from build123d import *

# Parameters (mm, degrees)
CROQUIS1_W              = 100
CROQUIS1_H              = 100
SALIENTE_EXTRUIR1_DEPTH = 12.5
CROQUIS3_R              = 35.2
CORTAR_EXTRUIR1_DEPTH   = 9.2
CROQUIS4_R              = 25.5
CORTAR_EXTRUIR2_DEPTH   = 72.30666168
CROQUIS5_R              = 3.25
CORTAR_EXTRUIR3_DEPTH   = 72.807033082
MATRIZC1_COUNT          = 4
CROQUIS6_R              = 5.5
CORTAR_EXTRUIR4_DEPTH   = 6
MATRIZC2_COUNT          = 4


with BuildPart() as part:
    # Croquis1 → Saliente-Extruir1 (new body)
    with BuildSketch(Plane(origin=(0, 0, 0), x_dir=(1, 0, 0), z_dir=(0, 1, 0))):
        Rectangle(CROQUIS1_W, CROQUIS1_H)
    extrude(amount=SALIENTE_EXTRUIR1_DEPTH)

    # Croquis3 → Cortar-Extruir1 (cut)
    with BuildSketch(Plane.XZ):
        with Locations(Location((0, 0, 0), (0, 0, 270))):
            Circle(CROQUIS3_R)
    extrude(amount=-CORTAR_EXTRUIR1_DEPTH, mode=Mode.SUBTRACT)

    # Croquis4 → Cortar-Extruir2 (cut, through all)
    with BuildSketch(Plane.XZ.offset(-9.2)):
        with Locations(Location((0, 0, 0), (0, 0, 270))):
            Circle(CROQUIS4_R)
    extrude(amount=-CORTAR_EXTRUIR2_DEPTH, mode=Mode.SUBTRACT)

    # Croquis5 → Cortar-Extruir3 (cut, through all)
    with BuildSketch(Plane.XZ):
        with Locations(Location((-40, 40, 0), (0, 0, 270))):
            Circle(CROQUIS5_R)
    cortar_extruir3 = extrude(amount=-CORTAR_EXTRUIR3_DEPTH, mode=Mode.SUBTRACT)

    # MatrizC1: Cortar-Extruir3 ×4 about axis
    matrizc1_axis = Axis((0, 0, 0), (0, 1, 0))
    for i in range(1, MATRIZC1_COUNT):
        add(cortar_extruir3.rotate(matrizc1_axis, i * 360 / MATRIZC1_COUNT), mode=Mode.SUBTRACT)

    # Croquis6 → Cortar-Extruir4 (cut)
    with BuildSketch(Plane(origin=(0, 12.5, 0), x_dir=(1, 0, 0), z_dir=(0, 1, 0))):
        with Locations(Location((-40, 40, 0), (0, 0, 270))):
            Circle(CROQUIS6_R)
    cortar_extruir4 = extrude(amount=-CORTAR_EXTRUIR4_DEPTH, mode=Mode.SUBTRACT)

    # MatrizC2: Cortar-Extruir4 ×4 about axis
    matrizc2_axis = Axis((0, 0, 0), (0, 1, 0))
    for i in range(1, MATRIZC2_COUNT):
        add(cortar_extruir4.rotate(matrizc2_axis, i * 360 / MATRIZC2_COUNT), mode=Mode.SUBTRACT)


solid = part.part
Check sheet for the modelled part. Datum: model origin and axes. Units: mm. A direction names the side the tool comes from. Round coordinates to 2 decimals unless told otherwise and drop trailing zeros. Write each loop counter-clockwise with the first axis right and the second up, starting at its lowest first coordinate (ties: lowest second). Pieces come first, ordered by that corner, then holes. Notation, with made-up numbers: (77.25, 69.5) -> (124.25, 69.5) arc R26 ccw to (124.25, 107.5) -> close; hole circle Ø6 at (-7.5, 34). An arc over 180 degrees is marked (long way). Answer as CSV lines item,"result". Start each with the question number.
1) Tool access check on faces 4 (the flat face through (-50, 6, 1)), 5 (the flat face through (18.4, 9.2, -18.1)), 6 (the cylindrical face through (39.758, 9.542, 45.495)). Record the directions out of +Z, -Z, +X, -X, +Y, -Y that give a thin tool (end or side, any length) a straight path to the whole face; none if there is none.
2) Material ranges on line 1 (Z direction, x = 40, y = 8.4); line 2 (X direction, y = 8.25, z = -1), recorded low to high. Write a range as from..to.
3) Go/stop test with flat-tipped pins: P1, Ø3.5, axis at x = -37.5, z = 39.5, coming from the +Y side; P2, Ø6, axis at x = -40, z = 40, coming from the -Y side. Record where each tip stops, or that it passes through.
4) Section check B-B on x = 0. Enter the section's corners in (y, z).
5) Section check C-C on x = -40. Enter the section's corners in (y, z).
6) Release check for a two-part mould opening along Z. For faces 1 (the flat face through (-34, 0, -12)), 2 (the flat face through (-1, 6, 50)), 3 (the cylindrical face through (-45.495, 9.542, 39.758)) record: pulls with the +Z half, pulls with the -Z half, needs draft (parallel to the pull), parting line crosses it, or undercut.
7) Section check A-A on z = -40. Enter the section's corners in (x, y).
8) Section check D-D on z = 0. Enter the section's corners in (x, y), and give its area (3 significant figures).
Found:
1,face 4,"+Z, -Z, -X, +Y, -Y"
1,face 5,"-Y"
1,face 6,"+Y"
2,line 1,"z = -50..-45.5, -34.5..34.5, 45.5..50"
2,line 2,"x = -50..-35.19, 35.19..50"
3,P1,"stops at y = 6.5"
3,P2,"passes through"
4,outline,"(0, -50) -> (12.5, -50) -> (12.5, -25.5) -> (9.2, -25.5) -> (9.2, -35.2) -> (0, -35.2) -> close; (0, 35.2) -> (9.2, 35.2) -> (9.2, 25.5) -> (12.5, 25.5) -> (12.5, 50) -> (0, 50) -> close"
5,outline,"(0, -50) -> (12.5, -50) -> (12.5, -45.5) -> (6.5, -45.5) -> (6.5, -43.25) -> (0, -43.25) -> close; (0, -36.75) -> (6.5, -36.75) -> (6.5, -34.5) -> (12.5, -34.5) -> (12.5, 34.5) -> (6.5, 34.5) -> (6.5, 36.75) -> (0, 36.75) -> close; (0, 43.25) -> (6.5, 43.25) -> (6.5, 45.5) -> (12.5, 45.5) -> (12.5, 50) -> (0, 50) -> close"
6,face 1,"needs draft"
6,face 2,"pulls with the +Z half"
6,face 3,"undercut"
7,outline,"(-50, 0) -> (-43.25, 0) -> (-43.25, 6.5) -> (-45.5, 6.5) -> (-45.5, 12.5) -> (-50, 12.5) -> close; (-36.75, 0) -> (36.75, 0) -> (36.75, 6.5) -> (34.5, 6.5) -> (34.5, 12.5) -> (-34.5, 12.5) -> (-34.5, 6.5) -> (-36.75, 6.5) -> close; (43.25, 0) -> (50, 0) -> (50, 12.5) -> (45.5, 12.5) -> (45.5, 6.5) -> (43.25, 6.5) -> close"
8,outline,"(-50, 0) -> (-35.2, 0) -> (-35.2, 9.2) -> (-25.5, 9.2) -> (-25.5, 12.5) -> (-50, 12.5) -> close; (25.5, 9.2) -> (35.2, 9.2) -> (35.2, 0) -> (50, 0) -> (50, 12.5) -> (25.5, 12.5) -> close"
8,area,"434 mm^2"
